Check sheet for the modelled part. Datum: model origin and axes. Units: mm. Round coordinates to 2 decimals unless told otherwise and drop trailing zeros. Write each loop counter-clockwise with the first axis right and the second up, starting at its lowest first coordinate (ties: lowest second). Pieces come first, ordered by that corner, then holes. Notation, with made-up numbers: (-19.75, -38.75) -> (-1.75, -38.75) arc R7 cw to (-1.75, -29.75) -> close; hole circle Ø4 at (-32.75, 20). An arc over 180 degrees is marked (long way). One line per item, written item: value. Start each with the question number.
```python
from build123d import *

# Parameters (mm, degrees)
SKETCH1_W           = 78.74
SKETCH1_H           = 73.66
SKETCH1_R           = 6.25
SKETCH1_W_2         = 50.67
SKETCH1_H_2         = 19.3
SKETCH1_W_3         = 12
SKETCH1_H_3         = 12
BOSS_EXTRUDE1_DEPTH = 5


with BuildPart() as part:
    # Sketch1 → Boss-Extrude1 (new body)
    with BuildSketch(Plane(origin=(0, 0, 0), x_dir=(1, 0, 0), z_dir=(0, 1, 0))):
        with Locations((8.206850447, -27.291358184)):
            Rectangle(SKETCH1_W, SKETCH1_H)
        with Locations(Location((34.676850447, -18.233358184, 0), (0, 0, 270))):
            Circle(SKETCH1_R, mode=Mode.SUBTRACT)
        with Locations((-1.888149553, -3.261358184)):
            Rectangle(SKETCH1_W_2, SKETCH1_H_2, mode=Mode.SUBTRACT)
        with Locations((34.857850447, -38.733358184)):
            Rectangle(SKETCH1_W_3, SKETCH1_H_3, mode=Mode.SUBTRACT)
        with Locations((34.857850447, -53.833358184)):
            Rectangle(SKETCH1_W_3, SKETCH1_H_3, mode=Mode.SUBTRACT)
    extrude(amount=BOSS_EXTRUDE1_DEPTH)


solid = part.part
```
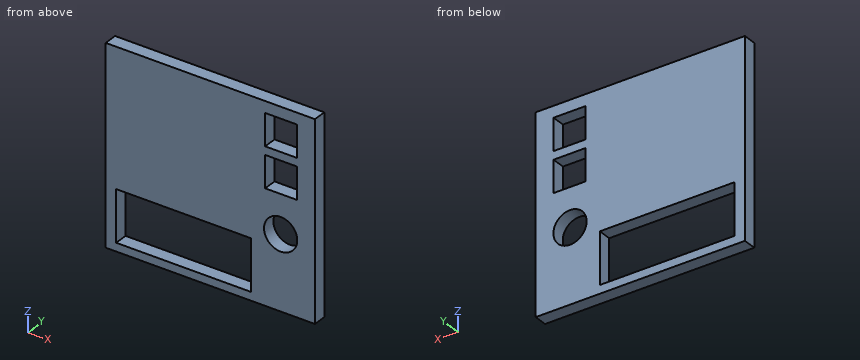
1. Material ranges on probe 1 along Z at (x, y) = (-24, 4.4); probe 2 along X at (y, z) = (3.95, -6); probe 3 along X at (y, z) = (1.95, 44.5), recorded low to high.
2. Cross-section at A-A (z = -0.5). Record the cut outline in (x, y), plus the area to 3 significant figures.
3. Cross-section at D-D (x = 32). Record the cut outline in (y, z).
4. Cross-section at B-B (x = 10.5). Record the cut outline in (y, z), plus the area to 3 significant figures.
5. Cross-section at C-C (y = 3.65). Record the cut outline in (x, z), plus the area to 3 significant figures.
Working result:
1. probe 1: z = -9.54 to -6.39, 12.91 to 64.12
1. probe 2: x = -31.16 to -27.22, 23.45 to 47.58
1. probe 3: x = -31.16 to 28.86, 40.86 to 47.58
2. outline: (-31.16, 0) -> (-27.22, 0) -> (-27.22, 5) -> (-31.16, 5) -> close; (23.45, 0) -> (47.58, 0) -> (47.58, 5) -> (23.45, 5) -> close
2. area: 140 mm^2
3. outline: (0, -9.54) -> (5, -9.54) -> (5, 12.59) -> (0, 12.59) -> close; (0, 23.88) -> (5, 23.88) -> (5, 32.73) -> (0, 32.73) -> close; (0, 44.73) -> (5, 44.73) -> (5, 47.83) -> (0, 47.83) -> close; (0, 59.83) -> (5, 59.83) -> (5, 64.12) -> (0, 64.12) -> close
4. outline: (0, -9.54) -> (5, -9.54) -> (5, -6.39) -> (0, -6.39) -> close; (0, 12.91) -> (5, 12.91) -> (5, 64.12) -> (0, 64.12) -> close
4. area: 272 mm^2
5. outline: (-31.16, -9.54) -> (47.58, -9.54) -> (47.58, 64.12) -> (-31.16, 64.12) -> close; hole (-27.22, -6.39) -> (23.45, -6.39) -> (23.45, 12.91) -> (-27.22, 12.91) -> close; hole circle Ø12.5 at (34.68, 18.23); hole (28.86, 32.73) -> (40.86, 32.73) -> (40.86, 44.73) -> (28.86, 44.73) -> close; hole (28.86, 47.83) -> (40.86, 47.83) -> (40.86, 59.83) -> (28.86, 59.83) -> close
5. area: 4,410 mm^2
